Read the model definition and answer for the solid it produces. Units are mm, in the model's axes. A direction names the side the tool comes from. Coordinates: 2 decimals unless noted, no trailing zeros. Order: outer loops, then holes, each group sorted by start corner. A loop starts at its lowest first (then second) coordinate and runs counter-clockwise, first axis right, second up. Notation, with made-up numbers: (30, 3) -> (78, 3) arc R35 ccw to (78, 36) -> close; hole circle Ø5 at (74, 48). An arc over 180 degrees is marked (long way). Answer as a JSON object with one key per item and string values. Group by question number.
1) Given pin 1 (1.5 mm diameter, centred on x = -2.5, z = 24, fed in from +Y); pin 2 (2 mm diameter, centred on x = 1, y = -31, fed in from +Z); pin 3 (1.5 mm diameter, centred on x = 1.5, z = 29.5, fed in from -Y); pin 4 (1.2 mm diameter, centred on x = 0.5, y = -2.5, fed in from +Z), each flat-ended and moving along its own axis, determine where each tip first touches the part or whether it passes through.
2) A tool of negligible diameter and unlimited length cuts with its end or side. For faces 1 (the cylindrical face through (6.215, -10.699, 28.028)), 2 (the cylindrical face through (-6.215, -3.301, 28.028)), 3 (the cylindrical face through (-6.215, -27.699, 9.726)), from which of +Z, -Z, +X, -X, +Y, -Y can it reach the whole face along a straight path? Write none if from no direction.
3) Section B-B on x = -2 is taken. Determine the outline of the cut face in (y, z), and give its area (3 significant figures).
4) Consider L1, parallel to Z at x = -5, y = -19.5; L2, parallel to X at y = -32, z = 19.85; L3, parallel to Y at x = 1.5, z = 27. Determine where each line is inside the solid, lowest interval first.
5) Determine the mould class of faces 4 (the flat face through (0, -29, 21)), 5 (the cylindrical face through (0.1, -29.5, 20)), 6 (the cylindrical face through (6.215, -33.699, 19.986)), 7 (the cylindrical face through (6.215, -0.301, 23.535)) for opening direction Y: released by +Y, released by -Y, zero draft, split by the parting line, or undercut.
6) Section A-A on y = 2.5 is taken. Determine the outline of the cut face in (x, z), and give its area (3 significant figures).
7) Section D-D on y = -7 is taken. Determine the outline of the cut face in (x, z), and give its area (3 significant figures).
8) Section C-C on z = 3.5 is taken. Determine the outline of the cut face in (x, y), and give its area (3 significant figures).
from build123d import *

# Parameters (mm, degrees)
F0_W     = 8
F0_H     = 4
F1_DEPTH = 6.5
F2_R     = 1.5
F3_DEPTH = 3
F4_SIZE  = 1
F5_R     = 1
F6_R     = 2.5
F7_DEPTH = 25


with BuildPart() as f1:
    # F0 (on Right) → F1 (new body, symmetric)
    with BuildSketch(Plane.YZ):
        Polygon((0, 0), (0, 19), (6, 19), (6, 21), (0, 21), (0, 26), (-3, 26), (-11, 26), (-28, 26), (-28, 21), (-34, 21), (-34, 19), (-28, 19), (-28, 0), align=None)
        with Locations((-7, 28)):
            Rectangle(F0_W, F0_H)
    extrude(amount=F1_DEPTH, both=True)

    # F2 (on face) → F3 (join)
    with BuildSketch(Plane.XY.offset(30)):
        with Locations((0, -7)):
            Circle(F2_R)
    extrude(amount=F3_DEPTH)

    # F4
    f4_edges = [f1.edges().sort_by_distance(p)[0] for p in [
        (-6.5, -14, 0),
        (0, 0, 0),
        (6.5, -14, 0),
        (0, -28, 0),
    ]]
    chamfer(f4_edges, length=F4_SIZE)

    # F5
    f5_edges = [f1.edges().sort_by_distance(p)[0] for p in [
        (6.5, 0, 10),
        (6.5, 0, 23.5),
        (-6.5, 0, 23.5),
        (6.5, -3, 28),
        (6.5, -11, 28),
        (-6.5, -11, 28),
        (-6.5, -3, 28),
        (6.5, -28, 23.5),
        (-6.5, -28, 23.5),
        (6.5, -34, 20),
        (-6.5, -34, 20),
        (6.5, -28, 10),
        (-6.5, -28, 10),
        (6.5, 6, 20),
        (-6.5, 6, 20),
    ]]
    fillet(f5_edges, radius=F5_R)

    # F6 (on face) → F7 (cut)
    with BuildSketch(Plane.XY.offset(21)):
        with Locations((0, 4)):
            Circle(F6_R)
        with Locations((0, -32)):
            Circle(F6_R)
    extrude(amount=-F7_DEPTH, mode=Mode.SUBTRACT)


solid = f1.part
Worked answers:
{
 "1": {"pin 1": "stops at y = 0", "pin 2": "passes through", "pin 3": "stops at y = -11", "pin 4": "stops at z = 30"},
 "2": {"face 1": "+Z, +X, -Y", "face 2": "+Z, -X, +Y", "face 3": "-Z, -X, -Y"},
 "3": {"outline": "(-34, 19) -> (-33.5, 19) -> (-33.5, 21) -> (-34, 21) -> close; (-30.5, 19) -> (-28, 19) -> (-28, 1) -> (-27, 0) -> (-1, 0) -> (0, 1) -> (0, 19) -> (2.5, 19) -> (2.5, 21) -> (0, 21) -> (0, 26) -> (-3, 26) -> (-3, 30) -> (-11, 30) -> (-11, 26) -> (-28, 26) -> (-28, 21) -> (-30.5, 21) -> close; (5.5, 19) -> (6, 19) -> (6, 21) -> (5.5, 21) -> close", "area": "771 mm²"},
 "4": {"L1": "z = 0 to 26", "L2": "x = -6.5 to -2.5, 2.5 to 6.5", "L3": "y = -11 to -3"},
 "5": {"face 4": "zero draft", "face 5": "undercut", "face 6": "released by -Y", "face 7": "released by +Y"},
 "6": {"outline": "(-6.5, 19) -> (-2, 19) -> (-2, 21) -> (-6.5, 21) -> close; (2, 19) -> (6.5, 19) -> (6.5, 21) -> (2, 21) -> close", "area": "18.0 mm²"},
 "7": {"outline": "(-6.5, 1) -> (-5.5, 0) -> (5.5, 0) -> (6.5, 1) -> (6.5, 30) -> (1.5, 30) -> (1.5, 33) -> (-1.5, 33) -> (-1.5, 30) -> (-6.5, 30) -> close", "area": "398 mm²"},
 "8": {"outline": "(-6.5, -27) arc R1 ccw to (-5.5, -28) -> (5.5, -28) arc R1 ccw to (6.5, -27) -> (6.5, -1) arc R1 ccw to (5.5, 0) -> (-6.5, 0) -> close", "area": "363 mm²"}
}
